Design review of the part built by this model. Coordinates are the model's own, in mm. A direction names the side the tool comes from. Round coordinates to 2 decimals unless told otherwise and drop trailing zeros. Write each loop counter-clockwise with the first axis right and the second up, starting at its lowest first coordinate (ties: lowest second). Pieces come first, ordered by that corner, then holes. Notation, with made-up numbers: M -21.75,79 L -5.75,79 A12 cw -5.75,90 Z; hole C 88,-28 d3. An arc over 180 degrees is marked long. One line per question, with ' | ' between items. Start each with the question number.
Item 1: Add section D-D, the plane y = 13.5. State the section outline as (x, z) points.
Item 2: Add section B-B, the plane x = -32.75. Give the number of separate pieces and of enclosed holes in the cut face, and give its area (3 significant figures).
Item 3: For L1, parallel to Y at x = -33, z = 10; L2, parallel to X at y = 43, z = 3.5, list the stretches that pass through material, from the lowest coordinate up.
Item 4: Insertion check: pin 1 Ø3.5 at (y, z) = (42.33, -9.83) entering from +X; pin 2 Ø5 at (x, y) = (23.5, 11.5) entering from +Z; pin 3 Ø12 at (y, z) = (25.5, 13.5) entering from +X. Each pin has a flat end and moves straight along its axis. Give the tip position at first contact, or say it passes through.
Item 5: Machinability: for faces 4 (the face through (-29, 3.93, -0.38)), 5 (the face through (-31.513, 1.232, -34.099)), 6 (the face through (-35.65, 27, 0)), 7 (the face through (-33.11, 39.11, 8.06)), 8 (the face through (23, 45.5, 0)), which of the approach directions +Z, -Z, +X, -X, +Y, -Y give a long, thin tool a straight path to every point of the face, cutting with its end or side? Answer none if there is none.
Item 6: Add section A-A, the plane z = -32.75. State the section outline as (x, y) points, and give its area (3 significant figures).
Item 7: Add section C-C, the plane x = 0. State the section outline as (y, z) points, and give its area (3 significant figures).
Item 8: Draft analysis for pull direction X (two halves, no side actions). For faces 1 (the face through (-31.513, 1.232, 31.401)), 2 (the face through (20, 32, 3)), 3 (the face through (23.35, 44.21, 16.65)), state which applies: released by +X, released by -X, zero draft, split by the parting line, or undercut.
```python
from build123d import *

# Parameters (mm, degrees)
SKETCH1_W           = 77.5
SKETCH1_H           = 77.5
SKETCH1_R           = 1.83
SKETCH1_R_2         = 13.5
BOSS_EXTRUDE1_DEPTH = 2.5
FILLET1_R           = 3
SKETCH2_W           = 5.15
SKETCH2_H           = 32
SKETCH2_W_2         = 3.65
BOSS_EXTRUDE2_DEPTH = 43
SKETCH3_R           = 3.875
SKETCH3_R_2         = 1.075
CUT_EXTRUDE1_DEPTH  = 10
SKETCH4_R           = 2.65
CUT_EXTRUDE2_DEPTH  = 10
SKETCH5_R           = 3.875
SKETCH5_R_2         = 2.65
BOSS_EXTRUDE3_DEPTH = 1.5
CHAMFER1_SIZE       = 1.5
CHAMFER2_SIZE       = 57.010424996
CHAMFER2_SIZE_2     = 7
CHAMFER3_SIZE       = 2
CHAMFER3_SIZE2      = 16.288692856
FILLET2_R           = 5


# Some blends are built 0.0001 mm under size
with BuildPart() as part:
    # Sketch1 → Boss-Extrude1 (new body)
    with BuildSketch(Plane(origin=(0, 0, 0), x_dir=(1, 0, 0), z_dir=(0, 1, 0))):
        Rectangle(SKETCH1_W, SKETCH1_H)
        with Locations(Location((32.75, 32.75, 0), (0, 0, 270))):
            Circle(SKETCH1_R, mode=Mode.SUBTRACT)
        with Locations(Location((32.75, -32.75, 0), (0, 0, 270))):
            Circle(SKETCH1_R, mode=Mode.SUBTRACT)
        with Locations(Location((-32.75, -32.75, 0), (0, 0, 270))):
            Circle(SKETCH1_R, mode=Mode.SUBTRACT)
        with Locations(Location((-32.75, 32.75, 0), (0, 0, 270))):
            Circle(SKETCH1_R, mode=Mode.SUBTRACT)
        with Locations(Location((0, 0, 0), (0, 0, 270))):
            Circle(SKETCH1_R_2, mode=Mode.SUBTRACT)
    extrude(amount=BOSS_EXTRUDE1_DEPTH)

    # Fillet1
    fillet1_edges = [part.edges().sort_by_distance(p)[0] for p in [
        (38.75, 1.25, 38.75),
        (-38.75, 1.25, 38.75),
        (-38.75, 1.25, -38.75),
        (38.75, 1.25, -38.75),
    ]]
    fillet(fillet1_edges, radius=FILLET1_R)

    # Sketch2 → Boss-Extrude2 (add)
    with BuildSketch(Plane(origin=(0, 2.5, 0), x_dir=(1, 0, 0), z_dir=(0, 1, 0))):
        with Locations((-33.075, 0)):
            Rectangle(SKETCH2_W, SKETCH2_H)
        with Locations((23.325, 0)):
            Rectangle(SKETCH2_W_2, SKETCH2_H)
    extrude(amount=BOSS_EXTRUDE2_DEPTH)

    # Sketch3 → Cut-Extrude1 (cut)
    with BuildSketch(Plane.ZY.offset(35.65)):
        with Locations((0, 32.5)):
            Circle(SKETCH3_R)
        with Locations((-5.303300859, 37.803300859)):
            Circle(SKETCH3_R_2)
        with Locations((5.303300859, 37.803300859)):
            Circle(SKETCH3_R_2)
        with Locations((5.303300859, 27.196699141)):
            Circle(SKETCH3_R_2)
        with Locations((-5.303300859, 27.196699141)):
            Circle(SKETCH3_R_2)
        with Locations((-7.566042559, 40.066042559)):
            Circle(SKETCH3_R_2)
        with Locations((-9.828784258, 42.328784258)):
            Circle(SKETCH3_R_2)
        with Locations((9.828784258, 42.328784258)):
            Circle(SKETCH3_R_2)
        with Locations((7.566042559, 40.066042559)):
            Circle(SKETCH3_R_2)
        with Locations((9.828784258, 22.671215742)):
            Circle(SKETCH3_R_2)
        with Locations((7.566042559, 24.933957441)):
            Circle(SKETCH3_R_2)
        with Locations((-9.828784258, 22.671215742)):
            Circle(SKETCH3_R_2)
        with Locations((-7.566042559, 24.933957441)):
            Circle(SKETCH3_R_2)
    extrude(amount=-CUT_EXTRUDE1_DEPTH, mode=Mode.SUBTRACT)

    # Sketch4 → Cut-Extrude2 (cut)
    with BuildSketch(Plane(origin=(25.15, 0, 0), x_dir=(0, 0, -1), z_dir=(1, 0, 0))):
        with Locations((0, 32.5)):
            Circle(SKETCH4_R)
    extrude(amount=-CUT_EXTRUDE2_DEPTH, mode=Mode.SUBTRACT)

    # Sketch5 → Boss-Extrude3 (add)
    with BuildSketch(Plane.ZY.offset(-21.5)):
        with Locations((0, 32.5)):
            Circle(SKETCH5_R)
        with Locations(Location((0, 32.5, 0), (0, 0, 180))):
            Circle(SKETCH5_R_2, mode=Mode.SUBTRACT)
    extrude(amount=BOSS_EXTRUDE3_DEPTH)

    # Chamfer1
    chamfer1_edges = [part.edges().sort_by_distance(p)[0] for p in [
        (21.5, 32.5, -3.875),
    ]]
    chamfer(chamfer1_edges, length=CHAMFER1_SIZE - 0.0001)  # a hair under: the kernel refuses the full size

    # Chamfer2
    # the kernel refuses this chamfer: 57.010424996, 7 mm, written as the material it adds along each edge
    with BuildSketch(Plane(origin=(25.15, 2.5, 16), x_dir=(0, 0.9999890085715016, -0.004688575069790725), z_dir=(-1, 0, 0))) as chamfer2_piece_1_section:
        Polygon((CHAMFER2_SIZE * 0.999989008568, -CHAMFER2_SIZE * 0.00468857506978), (-CHAMFER2_SIZE_2 * 0.00468857506979, -CHAMFER2_SIZE_2 * 0.999989008572), (0, 0), align=None)
    chamfer2_piece_1 = extrude(amount=3.65, mode=Mode.PRIVATE)
    chamfer2_piece_1 = split(chamfer2_piece_1, bisect_by=Plane(origin=(23.325, 45.5, 17.927649929), z_dir=(0, -1, 0)), keep=Keep.TOP, mode=Mode.PRIVATE)
    add(chamfer2_piece_1)
    with BuildSketch(Plane(origin=(25.15, 2.5, 16), x_dir=(0, 0.9999890085715016, -0.004688575069790725), z_dir=(-1, 0, 0))) as chamfer2_piece_2_section:
        Polygon((CHAMFER2_SIZE * 0.999989008568, -CHAMFER2_SIZE * 0.00468857506978), (-CHAMFER2_SIZE_2 * 0.00468857506979, -CHAMFER2_SIZE_2 * 0.999989008572), (0, 0), align=None)
    chamfer2_piece_2 = extrude(amount=151.836239061, mode=Mode.PRIVATE)
    chamfer2_piece_2 = split(chamfer2_piece_2, bisect_by=Plane(origin=(-33.075, 45.5, 17.927649929), z_dir=(0, -1, 0)), keep=Keep.TOP, mode=Mode.PRIVATE)
    chamfer2_piece_2 = split(chamfer2_piece_2, bisect_by=Plane(origin=(-35.65, 19.754331074, 17.927649929), z_dir=(1, 0, 0)), keep=Keep.TOP, mode=Mode.PRIVATE)
    chamfer2_piece_2 = split(chamfer2_piece_2, bisect_by=Plane(origin=(-30.5, 19.754331074, 17.927649929), z_dir=(-1, 0, 0)), keep=Keep.TOP, mode=Mode.PRIVATE)
    add(chamfer2_piece_2)
    with BuildSketch(Plane(origin=(117.686239061, 2.5, 16), x_dir=(0, -0.29696840376136574, 0.9548873060039212), z_dir=(-1, 0, 0))) as chamfer2_piece_3_section:
        Polygon((CHAMFER2_SIZE_2 * 0.954887306004, CHAMFER2_SIZE_2 * 0.296968403761), (-CHAMFER2_SIZE * 0.29696840376, CHAMFER2_SIZE * 0.954887306001), (0, 0), align=None)
    chamfer2_piece_3 = extrude(amount=153.336239061, mode=Mode.PRIVATE)
    chamfer2_piece_3 = split(chamfer2_piece_3, bisect_by=Plane(origin=(21.5, 19.754331074, 17.927649929), z_dir=(1, 0, 0)), keep=Keep.TOP, mode=Mode.PRIVATE)
    chamfer2_piece_3 = split(chamfer2_piece_3, bisect_by=Plane(origin=(25.15, 19.754331074, 17.927649929), z_dir=(-1, 0, 0)), keep=Keep.TOP, mode=Mode.PRIVATE)
    chamfer2_piece_3 = split(chamfer2_piece_3, bisect_by=Plane(origin=(23.325, 45.5, 17.927649929), z_dir=(0, -1, 0)), keep=Keep.TOP, mode=Mode.PRIVATE)
    add(chamfer2_piece_3)
    with BuildSketch(Plane(origin=(-30.5, 2.5, 16), x_dir=(0, -0.29696840376136574, 0.9548873060039212), z_dir=(-1, 0, 0))) as chamfer2_piece_4_section:
        Polygon((CHAMFER2_SIZE_2 * 0.954887306004, CHAMFER2_SIZE_2 * 0.296968403761), (-CHAMFER2_SIZE * 0.29696840376, CHAMFER2_SIZE * 0.954887306001), (0, 0), align=None)
    chamfer2_piece_4 = extrude(amount=5.15, mode=Mode.PRIVATE)
    chamfer2_piece_4 = split(chamfer2_piece_4, bisect_by=Plane(origin=(-33.075, 45.5, 17.927649929), z_dir=(0, -1, 0)), keep=Keep.TOP, mode=Mode.PRIVATE)
    add(chamfer2_piece_4)
    with BuildSketch(Plane(origin=(-35.65, 2.5, -16), x_dir=(0, -0.29696840376136574, -0.9548873060039212), z_dir=(1, 0, 0))) as chamfer2_piece_5_section:
        Polygon((CHAMFER2_SIZE_2 * 0.954887306004, CHAMFER2_SIZE_2 * 0.296968403761), (-CHAMFER2_SIZE * 0.29696840376, CHAMFER2_SIZE * 0.954887306001), (0, 0), align=None)
    chamfer2_piece_5 = extrude(amount=5.15, mode=Mode.PRIVATE)
    chamfer2_piece_5 = split(chamfer2_piece_5, bisect_by=Plane(origin=(-33.075, 45.5, -17.927649929), z_dir=(0, -1, 0)), keep=Keep.TOP, mode=Mode.PRIVATE)
    add(chamfer2_piece_5)
    with BuildSketch(Plane(origin=(-35.65, 2.5, -16), x_dir=(0, -0.29696840376136574, -0.9548873060039212), z_dir=(1, 0, 0))) as chamfer2_piece_6_section:
        Polygon((CHAMFER2_SIZE_2 * 0.954887306004, CHAMFER2_SIZE_2 * 0.296968403761), (-CHAMFER2_SIZE * 0.29696840376, CHAMFER2_SIZE * 0.954887306001), (0, 0), align=None)
    chamfer2_piece_6 = extrude(amount=153.336239061, mode=Mode.PRIVATE)
    chamfer2_piece_6 = split(chamfer2_piece_6, bisect_by=Plane(origin=(21.5, 19.754331074, -17.927649929), z_dir=(1, 0, 0)), keep=Keep.TOP, mode=Mode.PRIVATE)
    chamfer2_piece_6 = split(chamfer2_piece_6, bisect_by=Plane(origin=(23.325, 45.5, -17.927649929), z_dir=(0, -1, 0)), keep=Keep.TOP, mode=Mode.PRIVATE)
    chamfer2_piece_6 = split(chamfer2_piece_6, bisect_by=Plane(origin=(25.15, 19.754331074, -17.927649929), z_dir=(-1, 0, 0)), keep=Keep.TOP, mode=Mode.PRIVATE)
    add(chamfer2_piece_6)
    with BuildSketch(Plane(origin=(-126.686239061, 2.5, -16), x_dir=(0, -0.29696840376136574, -0.9548873060039212), z_dir=(1, 0, 0))) as chamfer2_piece_7_section:
        Polygon((CHAMFER2_SIZE_2 * 0.954887306004, CHAMFER2_SIZE_2 * 0.296968403761), (-CHAMFER2_SIZE * 0.29696840376, CHAMFER2_SIZE * 0.954887306001), (0, 0), align=None)
    chamfer2_piece_7 = extrude(amount=151.836239061, mode=Mode.PRIVATE)
    chamfer2_piece_7 = split(chamfer2_piece_7, bisect_by=Plane(origin=(-33.075, 45.5, -17.927649929), z_dir=(0, -1, 0)), keep=Keep.TOP, mode=Mode.PRIVATE)
    chamfer2_piece_7 = split(chamfer2_piece_7, bisect_by=Plane(origin=(-35.65, 19.754331074, -17.927649929), z_dir=(1, 0, 0)), keep=Keep.TOP, mode=Mode.PRIVATE)
    chamfer2_piece_7 = split(chamfer2_piece_7, bisect_by=Plane(origin=(-30.5, 19.754331074, -17.927649929), z_dir=(-1, 0, 0)), keep=Keep.TOP, mode=Mode.PRIVATE)
    add(chamfer2_piece_7)
    with BuildSketch(Plane(origin=(21.5, 2.5, -16), x_dir=(0, -0.29696840376136574, -0.9548873060039212), z_dir=(1, 0, 0))) as chamfer2_piece_8_section:
        Polygon((CHAMFER2_SIZE_2 * 0.954887306004, CHAMFER2_SIZE_2 * 0.296968403761), (-CHAMFER2_SIZE * 0.29696840376, CHAMFER2_SIZE * 0.954887306001), (0, 0), align=None)
    chamfer2_piece_8 = extrude(amount=3.65, mode=Mode.PRIVATE)
    chamfer2_piece_8 = split(chamfer2_piece_8, bisect_by=Plane(origin=(23.325, 45.5, -17.927649929), z_dir=(0, -1, 0)), keep=Keep.TOP, mode=Mode.PRIVATE)
    add(chamfer2_piece_8)

    # Chamfer3
    chamfer3_edges = [part.edges().sort_by_distance(p)[0] for p in [
        (-35.65, 2.5, 0),
        (25.15, 2.5, 0),
    ]]
    chamfer3_side = [part.faces().sort_by_distance(p)[0] for p in [
        (0, 2.5, 37.653984489),
    ]]
    chamfer(chamfer3_edges, length=CHAMFER3_SIZE, length2=CHAMFER3_SIZE2, reference=chamfer3_side[0])

    # Fillet2
    fillet2_edges = [part.edges().sort_by_distance(p)[0] for p in [
        (24.325, 2.5, -23),
        (-34.075, 2.5, -23),
        (-34.075, 2.5, 23),
        (24.325, 2.5, 23),
        (23.325, 45.5, 17.720263881),
        (-33.075, 45.5, 17.720263881),
        (-33.075, 45.5, -17.720263881),
        (23.325, 45.5, -17.720263881),
        (27.15, 2.5, 0),
        (-30.5, 2.5, 0),
        (21.5, 2.5, 0),
    ]]
    fillet(fillet2_edges, radius=FILLET2_R)


solid = part.part
```
Computed values:
1) outline: M -36.3,-21.65 L -30.5,-21.65 L -30.5,21.65 L -36.3,21.65 Z; M 21.5,-21.65 L 25.8,-21.65 L 25.8,21.65 L 21.5,21.65 Z
2) separate pieces: 3 | enclosed holes: 13 | area: 1,840 mm^2
3) L1: y = 0 to 21.61, 23.73 to 41.27, 43.39 to 45.5 | L2: x = -35.65 to -30.5, 21.5 to 25.15
4) pin 1: stops at x = 25.15 | pin 2: stops at z = 22.2 | pin 3: stops at x = 25.15
5) face 4: +Z, -Z, +Y | face 5: +Y, -Y | face 6: +Z, -Z, -X, +Y | face 7: -X | face 8: +Z, -Z, +X, -X, +Y
6) outline: M -38.75,0 L -34.58,0 L -34.58,2.5 L -38.75,2.5 Z; M -30.92,0 L 30.92,0 L 30.92,2.5 L -30.92,2.5 Z; M 34.58,0 L 38.75,0 L 38.75,2.5 L 34.58,2.5 Z | area: 175 mm^2
7) outline: M 0,-38.75 L 2.5,-38.75 L 2.5,-13.5 L 0,-13.5 Z; M 0,13.5 L 2.5,13.5 L 2.5,38.75 L 0,38.75 Z | area: 126 mm^2
8) face 1: undercut | face 2: released by -X | face 3: zero draft
